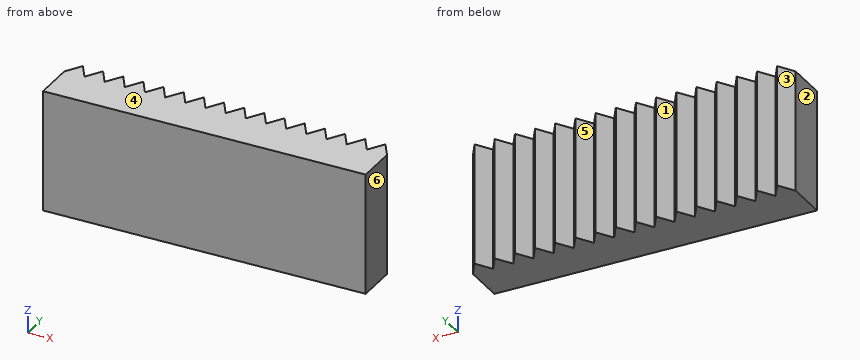
from build123d import *

# Parameters (mm, degrees)
BOSS_EXTRUDE1_DEPTH = 15


with BuildPart() as part:
    # Sketch1 → Boss-Extrude1 (new body)
    with BuildSketch(Plane.XY):
        Polygon((40, 0), (38.75, 2), (37.5, 0), (36.25, 2), (35, 0), (33.75, 2), (32.5, 0), (31.25, 2), (30, 0), (28.75, 2), (27.5, 0), (26.25, 2), (25, 0), (23.75, 2), (22.5, 0), (21.25, 2), (20, 0), (18.75, 2), (17.5, 0), (16.25, 2), (15, 0), (13.75, 2), (12.5, 0), (11.25, 2), (10, 0), (8.75, 2), (7.5, 0), (6.25, 2), (5, 0), (3.75, 2), (2.5, 0), (1.25, 2), (0, 0), (0, -5), (40, -5), align=None)
    extrude(amount=BOSS_EXTRUDE1_DEPTH)


solid = part.part
Here's how the part is built. I have some questions about the finished solid (model axes, mm). Face numbers are marked on the shaded views. A direction names the side the tool comes from. Give positions to 0.01 mm unless a question says otherwise; leave off trailing zeros. Loops run counter-clockwise (first coordinate to the right, second up) from the corner with the lowest first, then second, coordinate; pieces in that order, holes last. Notation, with made-up numbers: (71.5, 83) -> (110.5, 83) arc R31 ccw to (110.5, 116) -> close; hole circle Ø3 at (42.25, 25). An arc over 180 degrees is marked (long way). Answer as a JSON object with one key per item and string values. Group by question number.
Item 1: I need wall thicknesses on L1, parallel to Y at x = 18, z = 2; L2, parallel to Y at x = 36, z = 1.5. Which ranges of each line are inside material? Lowest first, please.
Item 2: Thinking about a two-plate mould opening in X: for the marked faces 3, 4, 5 and 6, which applies, pulls with the +X half, pulls with the -X half, needs draft (parallel to the pull), parting line crosses it, or undercut?
Item 3: Imagine slicing it at A-A on x = 32. Write out the boundary of the cut face in (y, z), then the cut area to 3 significant figures.
Item 4: On a 3-axis mill with a long thin cutter (end or side, diameter ignored), from which of +Z, -Z, +X, -X, +Y, -Y can I reach the whole of each face in a straight line? I mean the marked faces 1 and 2. Say none if no direction works.
Answer list:
{
 "1": {"L1": "y = -5 to 0.8", "L2": "y = -5 to 1.6"},
 "2": {"face 3": "pulls with the -X half", "face 4": "needs draft", "face 5": "undercut", "face 6": "pulls with the +X half"},
 "3": {"outline": "(-5, 0) -> (0.8, 0) -> (0.8, 15) -> (-5, 15) -> close", "area": "87.0 mm2"},
 "4": {"face 1": "+Z, -Z, +Y", "face 2": "+Z, -Z, -X, +Y, -Y"}
}
